Geometry check sheet. Reference: the model listing, model coordinates, mm. Face numbers are marked on the shaded views. A direction names the side the tool comes from. Give positions to 0.01 mm unless a question says otherwise; leave off trailing zeros. Loops run counter-clockwise (first coordinate to the right, second up) from the corner with the lowest first, then second, coordinate; pieces in that order, holes last. Notation, with made-up numbers: (88.25, 31.25) - (144.25, 31.25) arc R21 ccw to (144.25, 58.25) - close; hole circle Ø1 at (-37.5, 77). An arc over 180 degrees is marked (long way). Write item = value, one per line. Start each with the question number.
from build123d import *

# Parameters (mm, degrees)
SKETCH1_W             = 40
SKETCH1_H             = 84
SKETCH1_R             = 10.5
BOSS_EXTRUDE1_DEPTH   = 6
SKETCH2_W             = 40
SKETCH2_H             = 32
BOSS_EXTRUDE2_DEPTH   = 13
F_6_0MM_DOWEL_HOLE1_D = 6
M5_CLEARANCE_HOLE1_D  = 5.5
M4X0_7_TAPPED_HOLE1_D = 3.3
SKETCH12_R            = 17.5
CUT_EXTRUDE1_DEPTH    = 0.5
CUT_EXTRUDE2_START    = -0.5
SKETCH13_R            = 17.5
CUT_EXTRUDE2_DEPTH    = 0.5


with BuildPart() as part:
    # Sketch1 → Boss-Extrude1 (new body)
    with BuildSketch(Plane(origin=(0, 0, 0), x_dir=(1, 0, 0), z_dir=(0, 1, 0))):
        with Locations((0, -22)):
            Rectangle(SKETCH1_W, SKETCH1_H)
        with Locations(Location((0, 0, 0), (0, 0, 270))):
            Circle(SKETCH1_R, mode=Mode.SUBTRACT)
    extrude(amount=BOSS_EXTRUDE1_DEPTH)

    # Sketch2 → Boss-Extrude2 (add)
    with BuildSketch(Plane.XZ):
        with Locations((0, 48)):
            Rectangle(SKETCH2_W, SKETCH2_H)
    extrude(amount=BOSS_EXTRUDE2_DEPTH)

    # Ø6.0mm Dowel Hole1 (through all)
    with Locations(Plane(origin=(20, 0, 0), x_dir=(0, 0, -1), z_dir=(1, 0, 0))):
        with Locations((-57, -8), (-39, -8)):
            Hole(F_6_0MM_DOWEL_HOLE1_D / 2)

    # M5 Clearance Hole1 (through all)
    with Locations(Plane.ZY.offset(20)):
        with Locations((48, -8)):
            Hole(M5_CLEARANCE_HOLE1_D / 2)

    # M4x0.7 Tapped Hole1 (through all)
    with Locations(Plane(origin=(0, 0, 0), x_dir=(-1, 0, 0), z_dir=(0, -1, 0))):
        with Locations((16, 16), (-16, 16), (-16, -16), (16, -16)):
            Hole(M4X0_7_TAPPED_HOLE1_D / 2)

    # Sketch12 → Cut-Extrude1 (cut)
    with BuildSketch(Plane(origin=(0, 6, 0), x_dir=(1, 0, 0), z_dir=(0, 1, 0))):
        with Locations(Location((0, 0, 0), (0, 0, 270))):
            Circle(SKETCH12_R)
    extrude(amount=-CUT_EXTRUDE1_DEPTH, mode=Mode.SUBTRACT)

    # Sketch13 → Cut-Extrude2 (cut)
    with BuildSketch(Plane.XZ.offset(CUT_EXTRUDE2_START)):
        with Locations(Location((0, 0, 0), (0, 0, 90))):
            Circle(SKETCH13_R)
    extrude(amount=CUT_EXTRUDE2_DEPTH, mode=Mode.SUBTRACT)


solid = part.part
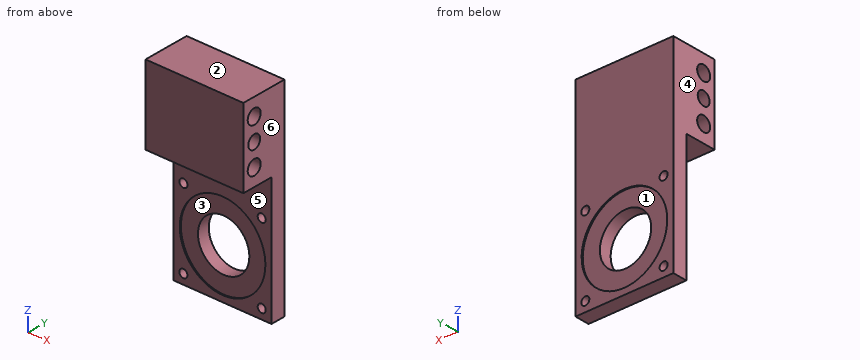
1) Cross-section at D-D on x = 15.5. Enter the section's corners in (y, z), and give its area (3 significant figures).
2) Tool access check on the marked faces 5 and 6. Record the directions out of +Z, -Z, +X, -X, +Y, -Y that give a thin tool (end or side, any length) a straight path to the whole face; none if there is none.
3) Cross-section at C-C on y = 3.75. Enter the section's corners in (x, z).
4) Cross-section at B-B on x = 0. Enter the section's corners in (y, z).
5) Release check for a two-part mould opening along X. For the marked faces 1, 2, 3 and 4 record: pulls with the +X half, pulls with the -X half, needs draft (parallel to the pull), parting line crosses it, or undercut.
6) Gauge pin test, flat ends, axial feed: P1, Ø5.5, axis at x = 16, z = -16, coming from the -Y side; P2, Ø12, axis at x = -9, z = -6.5, coming from the -Y side; P3, Ø4.5, axis at x = -16, z = 16, coming from the +Y side; P4, Ø3, axis at x = -13.5, y = -8, coming from the -Z side. Record the tip position at first contact, or that the pin passes through.
7) Material ranges on line 1 along Z through (x, y) = (-16, 2.95); line 2 along X through (y, z) = (4.25, -16); line 3 along X through (y, z) = (5.8, 0), recorded low to high.
8) Cross-section at A-A on z = 48. Enter the section's corners in (x, y), and give its area (3 significant figures).
Checked values:
q1.outline = (-13, 32) - (0, 32) - (0, 17.57) - (6, 17.57) - (6, 64) - (-13, 64) - close; (0, -20) - (6, -20) - (6, -17.57) - (0, -17.57) - close; (0, -14.43) - (6, -14.43) - (6, -8.12) - (5.5, -8.12) - (5.5, 8.12) - (6, 8.12) - (6, 14.43) - (0, 14.43) - (0, 8.12) - (0.5, 8.12) - (0.5, -8.12) - (0, -8.12) - close; hole circle Ø6 at (-8, 39); hole circle Ø6 at (-8, 57); hole circle Ø5.5 at (-8, 48)
q1.area = 786 mm²
q2.face_5 = -Z, +X, -X, -Y
q2.face_6 = +Z, -Z, +X, +Y, -Y
q3.outline = (-20, -20) - (20, -20) - (20, 64) - (-20, 64) - close; hole circle Ø3.3 at (-16, -16); hole circle Ø3.3 at (-16, 16); hole circle Ø21 at (0, 0); hole circle Ø3.3 at (16, -16); hole circle Ø3.3 at (16, 16)
q4.outline = (-13, 32) - (0, 32) - (0, 17.5) - (0.5, 17.5) - (0.5, 10.5) - (5.5, 10.5) - (5.5, 17.5) - (6, 17.5) - (6, 64) - (-13, 64) - close; (0, -20) - (6, -20) - (6, -17.5) - (5.5, -17.5) - (5.5, -10.5) - (0.5, -10.5) - (0.5, -17.5) - (0, -17.5) - close; hole circle Ø6 at (-8, 39); hole circle Ø6 at (-8, 57); hole circle Ø5.5 at (-8, 48)
q5.face_1 = undercut
q5.face_2 = needs draft
q5.face_3 = undercut
q5.face_4 = pulls with the -X half
q6.P1 = 0
q6.P2 = 0.5
q6.P3 = 6
q6.P4 = 32
q7.line_1 = -20 to -17.65, -14.35 to 14.35, 17.65 to 64
q7.line_2 = -20 to -17.65, -14.35 to 14.35, 17.65 to 20
q7.line_3 = -20 to -17.5, 17.5 to 20
q8.outline = (-20, -13) - (20, -13) - (20, -10.75) - (-20, -10.75) - close; (-20, -5.25) - (20, -5.25) - (20, 6) - (-20, 6) - close
q8.area = 540 mm²
